Read the model definition and answer for the solid it produces. Units are mm, in the model's axes. Face numbers are marked on the shaded views. A direction names the side the tool comes from. Coordinates: 2 decimals unless noted, no trailing zeros. Write each loop counter-clockwise with the first axis right and the second up, starting at its lowest first coordinate (ties: lowest second). Pieces come first, ordered by that corner, then holes.
(1) The part is cut by section D-D, the plane y = -46. Determine the outline of the cut face in (x, z).
(2) Determine the mould class of the marked faces 6, 7 and 8 for opening direction Y: pulls with the +Y half, pulls with the -Y half, needs draft (parallel to the pull), parting line crosses it, or undercut.
(3) The part is cut by section C-C, the plane z = 16. Determine the outline of the cut face in (x, y), and give its area (3 significant figures).
(4) Given pin 1 (5 mm diameter, centred on x = -42, z = 22, fed in from +Y); pin 2 (1.5 mm diameter, centred on y = -41, z = 33, fed in from +X); pin 3 (14 mm diameter, centred on x = 14, z = 6, fed in from -Y), each flat-ended and moving along its own axis, determine where each tip first touches the part or whether it passes through.
(5) The part is cut by section B-B, the plane x = 60. Determine the outline of the cut face in (y, z), and give its area (3 significant figures).
(6) Which of the six approach directions +Z, -Z, +X, -X, +Y, -Y give full straight-line access (tool end or side, diameter ignored) to the marked faces 1, 2, 3, 4 and 5?
(7) The part is cut by section A-A, the plane y = 0. Determine the outline of the cut face in (x, z), and give its area (3 significant figures).
(8) Straight lines are drawn through the part: line 1 along Y through (x, z) = (61, 46); line 2 along Y through (x, z) = (45, 7); line 3 along X through (y, z) = (-15, 48). For each, find the intervals that lie inside material, in ascending order.
```python
from build123d import *

# Parameters (mm, degrees)
F0_W      = 121.971261
F0_H      = 116.605956
F1_DEPTH  = 12.7
F2_R      = 54.989942
F3_DEPTH  = 50.8
F4_R      = 38.676946
F5_DEPTH  = 101.6
F7_DEPTH  = 25.4
F9_DEPTH  = 50.8
F10_W     = 121.971261
F10_H     = 6.011137
F11_DEPTH = 25.4
F12_W     = 121.971261
F12_H     = 5.653453
F13_DEPTH = 25.4


with BuildPart() as f1:
    # F0 (on Top) → F1 (new body)
    with BuildSketch(Plane.XY):
        with Locations((-15.559384, -0.178842)):
            Rectangle(F0_W, F0_H)
    extrude(amount=F1_DEPTH)

    # F2 (on Top) → F3 (join)
    with BuildSketch(Plane.XY):
        with Locations((61.879851, 0)):
            Circle(F2_R)
    extrude(amount=F3_DEPTH)

    # F4 (on face) → F5 (cut)
    with BuildSketch(Plane.XY.offset(50.8)):
        with Locations((61.879851, 0)):
            Circle(F4_R)
    extrude(amount=-F5_DEPTH, mode=Mode.SUBTRACT)

    # F6 (on face) → F7 (join)
    with BuildSketch(Plane.XY.offset(12.7)):
        with BuildLine():
            ThreePointArc((8.404423, -12.816874), (6.889909, 0), (8.404423, 12.816874))
            Line((8.404423, 12.816874), (-64.918965, 12.816874))
            Line((-64.918965, 12.816874), (-64.918965, -12.816874))
            Line((-64.918965, -12.816874), (8.404423, -12.816874))
        make_face()
    extrude(amount=F7_DEPTH)

    # F8 (on face) → F9 (cut)
    with BuildSketch(Plane.XZ.offset(12.816874)):
        Polygon((-64.918965, 12.7), (8.404423, 38.1), (-64.918965, 38.1), align=None)
    extrude(amount=-F9_DEPTH, mode=Mode.SUBTRACT)

    # F10 (on face) → F11 (cut)
    with BuildSketch(Plane.XY.offset(12.7)):
        with Locations((-15.559384, -55.476252)):
            Rectangle(F10_W, F10_H)
    extrude(amount=-F11_DEPTH, mode=Mode.SUBTRACT)

    # F12 (on face) → F13 (cut)
    with BuildSketch(Plane.XY.offset(12.7)):
        with Locations((-15.559384, 55.29741)):
            Rectangle(F12_W, F12_H)
    extrude(amount=-F13_DEPTH, mode=Mode.SUBTRACT)


solid = f1.part
```
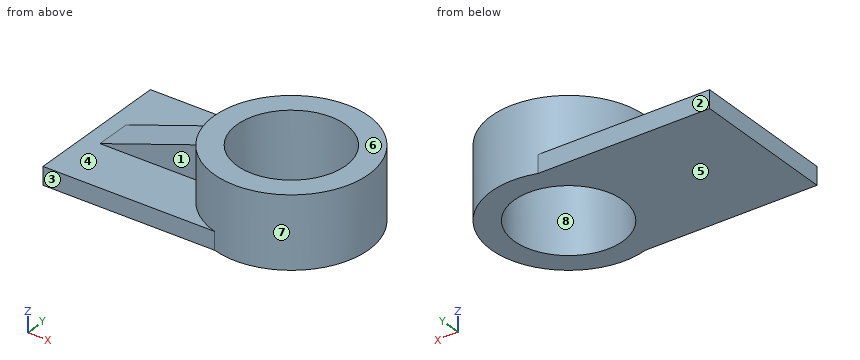
Computed:
1. outline: (-76.55, 0) - (92.01, 0) - (92.01, 50.8) - (31.75, 50.8) - (31.75, 12.7) - (-76.55, 12.7) - close
2. face 6: needs draft
2. face 7: parting line crosses it
2. face 8: undercut
3. outline: (-55.39, -12.82) - (8.4, -12.82) arc R54.99 ccw (long way) to (8.4, 12.82) - (-55.39, 12.82) - close; hole circle Ø77.35 at (61.88, 0)
3. area: 6,410 mm2
4. pin 1: stops at y = 12.82
4. pin 2: stops at x = 99.35
4. pin 3: stops at y = -52.47
5. outline: (-54.96, 0) - (-38.63, 0) - (-38.63, 50.8) - (-54.96, 50.8) - close; (38.63, 0) - (54.96, 0) - (54.96, 50.8) - (38.63, 50.8) - close
5. area: 1,660 mm2
6. face 1: +Z, -X, -Y
6. face 2: +Z, -Z, -X, +Y
6. face 3: +Z, -Z, -X, -Y
6. face 4: +Z, -X
6. face 5: -Z, +X, -X, +Y, -Y
7. outline: (-76.55, 0) - (23.2, 0) - (23.2, 50.8) - (6.89, 50.8) - (6.89, 38.1) - (8.4, 38.1) - (-64.92, 12.7) - (-76.55, 12.7) - close; (100.56, 0) - (116.87, 0) - (116.87, 50.8) - (100.56, 50.8) - close
7. area: 3,610 mm2
8. line 1: y = -54.98 to -38.67, 38.67 to 54.98
8. line 2: y = -52.47 to -34.8, 34.8 to 52.47
8. line 3: x = 8.98 to 26.23, 97.53 to 114.78
